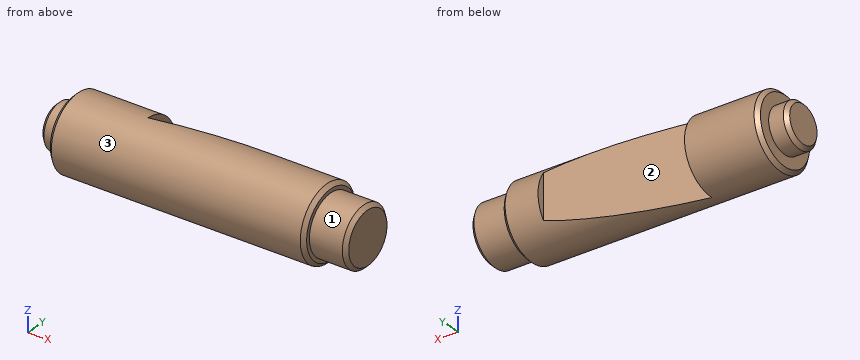
Autodesk Inventor part; units mm, degrees
ref_plane "YZ Plane" through (0, 0, 0) normal (1, 0, 0) x (0, 1, 0)
ref_plane "XZ Plane" through (0, 0, 0) normal (0, 1, 0) x (-1, 0, 0)
ref_plane "XY Plane" through (0, 0, 0) normal (0, 0, 1) x (1, 0, 0)
sketch "草图1" plane through (0, 0, 0) normal (0, 0, 1) x (1, 0, 0)
  line L0 (0, 0) -> (5, 0)
  line L1 (5, 0) -> (5, -6)
  line L2 (5, -6) -> (0, -6)
  line L3 (0, -6) -> (0, 0)
  line L4 (5, 0) -> (75, 0)
  line L5 (75, 0) -> (75, -10)
  line L6 (75, -10) -> (5, -10)
  line L7 (5, -10) -> (5, 0)
  line L8 (75, 0) -> (85, 0)
  line L9 (85, 0) -> (85, -8)
  line L10 (85, -8) -> (75, -8)
  line L11 (75, -8) -> (75, 0)
  dimension "d0" = 5
  dimension "d1" = 6
  dimension "d2" = 70
  dimension "d3" = 10
  dimension "d4" = 10
  dimension "d5" = 8
revolve "旋转1" add sketch "草图1" angle 360 about axis through (5, 0, 0) along (1, 0, 0)
sketch "草图2" plane through (0, 0, 0) normal (0, 0, 1) x (1, 0, 0)
  line L0 (5, 6) -> (0, 6)
  line L1 (0, 6) -> (0, -6)
  line L2 (1, 6) -> (0, 6)
  line L3 (0, 6) -> (0, 5)
  line L4 (1, 6) -> (0, 5)
  line L5 (1, 6) -> (0, 5)
  line L6 (5, 10) -> (5, -10)
  line L7 (5, 10) -> (6, 10)
  line L8 (6, 10) -> (6, 9)
  line L9 (6, 9) -> (5, 9)
  line L10 (5, 9) -> (5, 10)
  line L11 (5, 10) -> (5, 9)
  line L12 (84, 8) -> (84, 7)
  line L13 (84, 7) -> (85, 7)
  line L14 (85, 8) -> (85, -8)
  line L15 (85, 8) -> (85, 7)
  line L16 (75, 10) -> (75, -10)
  line L17 (75, 10) -> (74, 10)
  line L18 (74, 10) -> (74, 9)
  line L19 (74, 9) -> (75, 9)
  line L20 (75, 9) -> (75, 10)
  line L21 (75, 9) -> (74, 10)
  line L22 (75, 10) -> (75, 9)
  line L23 (85, 8) -> (84, 8)
  line L24 (84, 8) -> (84, 7)
  line L25 (84, 7) -> (85, 7)
  line L26 (85, 7) -> (85, 8)
  line L27 (85, 7) -> (84, 8)
  line L28 (85, 8) -> (85, 7)
  line L29 (6, 10) -> (5, 9)
  line L30 (-17, 0) -> (102, 0)
  point P0 (0, 0)
  dimension "d7" = 1
  dimension "d8" = 1
  dimension "d9" = 1
  dimension "d10" = 1
  dimension "d13" = 1
  dimension "d14" = 1
  dimension "d15" = 1
  dimension "d16" = 1
revolve "旋转2" cut sketch "草图2" angle 360 about axis through (-10, 0, 0) along (1, 0, 0) contours L6 L7 L29 | L21 L17 L16 | L27 L23 L14 | L4 L1 L0
sketch "草图3" plane through (0, 0, 0) normal (0, 0, 1) x (1, 0, 0)
  line L0 (74, 10) -> (6, 10)
  line L1 (75, 8) -> (75, -8)
  line L2 (65, 10) -> (65, 8)
  line L3 (74, 10) -> (74, -10)
  line L4 (25, 10) -> (25, 0)
  line L5 (5, 9) -> (5, -9)
  line L6 (25, 0) -> (65, 8)
  line L7 (65, 10) -> (25, 10)
  point P0 (0, 0)
  dimension "d18" = 10
  dimension "d19" = 2
  dimension "d20" = 10
  dimension "d21" = 20
extrude "拉伸1" cut sketch "草图3" along normal through all both and the other way through all
properties part number "9-滑轴" material "不锈钢"
Read the model definition and answer for the solid it produces. Units are mm, in the model's axes. Face numbers are marked on the shaded views. A direction names the side the tool comes from. Coordinates: 2 decimals unless noted, no trailing zeros. Write each loop counter-clockwise with the first axis right and the second up, starting at its lowest first coordinate (ties: lowest second). Pieces come first, ordered by that corner, then holes. Notation, with made-up numbers: (66, -14.75) -> (75, -14.75) arc R6 cw to (75, -8.75) -> close; hole circle Ø3 at (9.25, 74). An arc over 180 degrees is marked (long way). Answer as a JSON object with one key per item and string values.
Q1. Flat-ended cylindrical pins translate along their axes: pin 1 Ø8 at (y, z) = (-5.5, -7.5) entering from -X; pin 2 Ø1.5 at (x, y) = (17.5, -1) entering from +Z; pin 3 Ø2 at (x, y) = (22.5, 7.5) entering from +Z. Find the tip coordinate at first contact, or state that the pin passes through.
The answers:
{"pin 1": "stops at x = 0.3", "pin 2": "stops at z = 10", "pin 3": "stops at z = 7.6"}
Q2. The part is cut by section B-B on x = 20.5. Give the vertices of the cut face in (y, z), then the cut area to 3 significant figures.
The answers:
{"outline": "circle Ø20 at (0, 0)", "area": "314 mm2"}
Q3. The part is cut by section C-C on x = 37. Give the vertices of the cut face in (y, z).
The answers:
{"outline": "(2.4, -9.71) -> (2.4, 9.71) arc R10 ccw (long way) to start"}
Q4. Consider line 1 (X direction, y = -1, z = -8); line 2 (X direction, y = -1.75, z = -6); line 3 (Z direction, x = 53, y = -8). Determine where each line is inside the solid, lowest interval first. Write a range as [from, to].
The answers:
{"line 1": "x = [5, 75]", "line 2": "x = [5, 85]", "line 3": "z = [-6, 6]"}
Q5. The part is cut by section A-A on z = 0. Give the vertices of the cut face in (x, y), then the cut area to 3 significant figures.
The answers:
{"outline": "(0, -5) -> (1, -6) -> (5, -6) -> (5, -9) -> (6, -10) -> (74, -10) -> (75, -9) -> (75, -8) -> (84, -8) -> (85, -7) -> (85, 7) -> (84, 8) -> (75, 8) -> (75, 9) -> (74, 10) -> (65, 10) -> (65, 8) -> (25, 0) -> (25, 10) -> (6, 10) -> (5, 9) -> (5, 6) -> (1, 6) -> (0, 5) -> close", "area": "1,380 mm2"}
Q6. A tool of negligible diameter and unlimited length cuts with its end or side. For the marked faces 1, 2 and 3, from which of +Z, -Z, +X, -X, +Y, -Y can it reach the whole face along a straight path? Write none if from no direction.
The answers:
{"face 1": "+X", "face 2": "+Z, -Z, +Y", "face 3": "+X, -X"}
